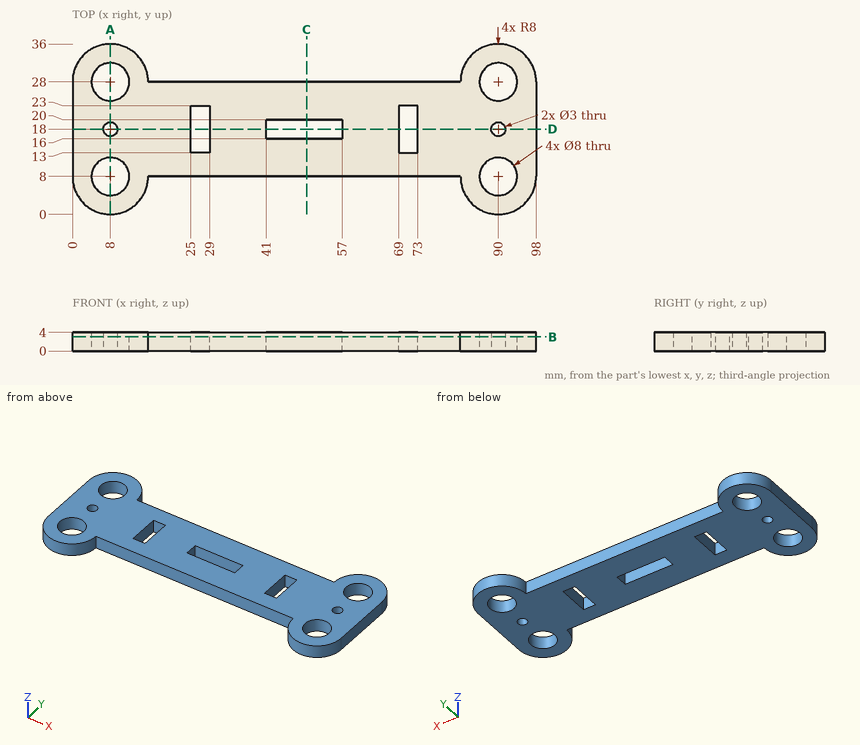
Study the drawing (mm; zero at the part's minimum x, y, z) and answer. Coordinates: 2 decimals unless noted, no trailing zeros. Write each loop counter-clockwise with the first axis right and the second up, starting at its lowest first coordinate (ties: lowest second). Pieces come first, ordered by that corner, then holes. Notation, with made-up numbers: (23, 31.25) -> (58, 31.25) arc R29 ccw to (58, 54.25) -> close; hole circle Ø4 at (-34, -5.75). An arc over 180 degrees is marked (long way). Write item = value, one per line.
(1) Given pin 1 Ø1.2 at (x, z) = (71, 1) entering from -Y; pin 2 Ø1 at (x, z) = (58.5, 3.5) entering from +Y, each flat-ended and moving along its own axis, determine where each tip first touches the part or whether it passes through.
From the geometry:
pin_1 = 8
pin_2 = 28
(2) Straight lines are drawn through the part: L1, parallel to Y at x = 90, z = 1.4; L2, parallel to X at y = 18, z = 1.95; L3, parallel to X at y = 15.5, z = 0.3. For each, find the intervals that lie inside material, in ascending order. Write a range as from..to.
From the geometry:
L1 = 0..4, 12..16.5, 19.5..24, 32..36
L2 = 0..6.5, 9.5..25, 29..41, 57..69, 73..88.5, 91.5..98
L3 = 0..25, 29..69, 73..98
(3) Section C-C on x = 49.5 is taken. Write down the section's boundary in (y, z), plus the area to 3 significant figures.
From the geometry:
outline = (8, 0) -> (16, 0) -> (16, 4) -> (8, 4) -> close; (20, 0) -> (28, 0) -> (28, 4) -> (20, 4) -> close
area = 64.0 mm2
(4) Section A-A on x = 8 is taken. Write down the section's boundary in (y, z), plus the area to 3 significant figures.
From the geometry:
outline = (0, 0) -> (4, 0) -> (4, 4) -> (0, 4) -> close; (12, 0) -> (16.5, 0) -> (16.5, 4) -> (12, 4) -> close; (19.5, 0) -> (24, 0) -> (24, 4) -> (19.5, 4) -> close; (32, 0) -> (36, 0) -> (36, 4) -> (32, 4) -> close
area = 68.0 mm2
(5) Section B-B on z = 3.05 is taken. Count the separate pieces of the cut face and the enclosed holes in it, plus the area to 3 significant figures.
From the geometry:
separate_pieces = 1
enclosed_holes = 9
area = 2,000 mm2
(6) Section D-D on y = 18 is taken. Write down the section's boundary in (x, z), plus the area to 3 significant figures.
From the geometry:
outline = (0, 0) -> (6.5, 0) -> (6.5, 4) -> (0, 4) -> close; (9.5, 0) -> (25, 0) -> (25, 4) -> (9.5, 4) -> close; (29, 0) -> (41, 0) -> (41, 4) -> (29, 4) -> close; (57, 0) -> (69, 0) -> (69, 4) -> (57, 4) -> close; (73, 0) -> (88.5, 0) -> (88.5, 4) -> (73, 4) -> close; (91.5, 0) -> (98, 0) -> (98, 4) -> (91.5, 4) -> close
area = 272 mm2
